Geometry: final body of the model. Coordinates: model frame, mm. A direction names the side the tool comes from. Give positions to 0.01 mm unless a question says otherwise; leave off trailing zeros. Order: outer loops, then holes, each group sorted by start corner. A loop starts at its lowest first (then second) coordinate and runs counter-clockwise, first axis right, second up. Notation, with made-up numbers: (21, 53) - (29, 53) arc R19 cw to (29, 64) - close; hole circle Ø6 at (19, -40). An arc over 180 degrees is marked (long way). One line per item, written item: value.
Autodesk Inventor part; units mm, degrees
ref_plane "YZ Plane" through (0, 0, 0) normal (1, 0, 0) x (0, 1, 0)
ref_plane "XZ Plane" through (0, 0, 0) normal (0, 1, 0) x (-1, 0, 0)
ref_plane "XY Plane" through (0, 0, 0) normal (0, 0, 1) x (1, 0, 0)
sketch "Эскиз1" plane through (0, 0, 0) normal (0, 1, 0) x (-1, 0, 0)
  line L0 (2.8868, 0) -> (1.4434, -2.5)
  line L1 (1.4434, -2.5) -> (-1.4434, -2.5)
  line L2 (-1.4434, -2.5) -> (-2.8868, 0)
  line L3 (-2.8868, 0) -> (-1.4434, 2.5)
  line L4 (-1.4434, 2.5) -> (1.4434, 2.5)
  line L5 (1.4434, 2.5) -> (2.8868, 0)
  point P0 (0, 0)
  point P1 (0, 0)
  dimension "d0" = 5
extrude "Выдавливание1" add sketch "Эскиз1" along normal blind 6
sketch "Эскиз2" plane through (0, 0, 0) normal (0, -1, 0) x (1, 0, 0)
  circle A0 centre (0, 0) radius 1.4
  dimension "d3" = 2.8
extrude "Выдавливание2" add sketch "Эскиз2" along normal blind 6
sketch "Эскиз3" plane through (0, 6, 0) normal (0, 1, 0) x (1, 0, 0)
  circle A0 centre (0, 0) radius 1.4
  dimension "d6" = 2.8
extrude "Выдавливание3" cut sketch "Эскиз3" against normal blind 5.6
thread "Резьба1"
thread "Резьба2"
properties part number "M3_MF_6mm"
1) Material intervals for line 1 along Z through (x, y) = (0, 2.5); line 2 along Y through (x, z) = (2.15, -0.85); line 3 along Z through (x, y) = (1.25, 2), sorted ascending.
Answers below:
line 1: -2.5 to -1.4, 1.4 to 2.5
line 2: 0 to 6
line 3: -2.5 to -0.63, 0.63 to 2.5
2) Section C-C, the plane z = 1.1. Return loops of the section in (x, y).
Answers below:
outline: (-2.25, 0) - (-0.87, 0) - (-0.87, -6) - (0.87, -6) - (0.87, 0) - (2.25, 0) - (2.25, 6) - (0.87, 6) - (0.87, 0.4) - (-0.87, 0.4) - (-0.87, 6) - (-2.25, 6) - close
3) Section A-A, the plane y = 2.75. Return loops of the section in (x, z), then the cut area to 3 significant figures.
Answers below:
outline: (-2.89, 0) - (-1.44, -2.5) - (1.44, -2.5) - (2.89, 0) - (1.44, 2.5) - (-1.44, 2.5) - close; hole circle Ø2.8 at (0, 0)
area: 15.5 mm^2
4) First-contact query: pin 1 (1 mm diameter, centred on x = 0, y = -2, fed in from -Z). Flat tip, straight axial feed; report the tip coordinate or a pass-through.
Answers below:
pin 1: z = -1.4
5) Mould query, pull axis X, two halves, no side actions, for faces 1 (the face through (-2.175, 2.958, -1.233)), 2 (the face through (-1.4, 3.24, -0.06)), 3 (the face through (-1.2, 0, 1.1)). Classes: released by +X, released by -X, zero draft, split by the parting line, or undercut.
Answers below:
face 1: released by -X
face 2: undercut
face 3: zero draft
6) Section B-B, the plane x = 0. Return loops of the section in (y, z), then the cut area to 3 significant figures.
Answers below:
outline: (-6, -1.4) - (0, -1.4) - (0, -2.5) - (6, -2.5) - (6, -1.4) - (0.4, -1.4) - (0.4, 1.4) - (6, 1.4) - (6, 2.5) - (0, 2.5) - (0, 1.4) - (-6, 1.4) - close
area: 31.1 mm^2
7) Set-up query: faces 4 (the face through (2.175, 2.958, 1.233)), 5 (the face through (0, 0.4, 0)), 6 (the face through (-1.4, -2.96, -0.06)). Return all of +Z, -Z, +X, -X, +Y, -Y with unobstructed straight access to the full face (end or side cutting, diameter ignored); none if empty.
Answers below:
face 4: +Z, +X, +Y, -Y
face 5: +Y
face 6: -Y
8) Section D-D, the plane z = -1.75. Return loops of the section in (x, y), then the cut area to 3 significant figures.
Answers below:
outline: (-1.88, 0) - (1.88, 0) - (1.88, 6) - (-1.88, 6) - close
area: 22.5 mm^2
